```python
from build123d import *

# Parameters (mm, degrees)
SKETCH1_R           = 7
SKETCH1_R_2         = 4
BOSS_EXTRUDE1_DEPTH = 300
SKETCH2_R           = 5
CUT_EXTRUDE1_DEPTH  = 31
CUT_EXTRUDE2_START  = -269
SKETCH2_2_R         = 5
CUT_EXTRUDE2_DEPTH  = 31


with BuildPart() as part:
    # Sketch1 → Boss-Extrude1 (new body)
    with BuildSketch(Plane(origin=(0, 0, 0), x_dir=(1, 0, 0), z_dir=(0, 1, 0))):
        with Locations(Location((0, 0, 0), (0, 0, 270))):
            Circle(SKETCH1_R)
        with Locations(Location((0, 0, 0), (0, 0, 270))):
            Circle(SKETCH1_R_2, mode=Mode.SUBTRACT)
    extrude(amount=BOSS_EXTRUDE1_DEPTH)

    # Sketch2 → Cut-Extrude1 (cut)
    with BuildSketch(Plane(origin=(0, 300, 0), x_dir=(1, 0, 0), z_dir=(0, 1, 0))):
        with Locations(Location((0, 0, 0), (0, 0, 270))):
            Circle(SKETCH2_R)
    extrude(amount=-CUT_EXTRUDE1_DEPTH, mode=Mode.SUBTRACT)

    # Sketch2<2> → Cut-Extrude2 (cut)
    with BuildSketch(Plane(origin=(0, 300, 0), x_dir=(1, 0, 0), z_dir=(0, 1, 0)).offset(CUT_EXTRUDE2_START)):
        with Locations(Location((0, 0, 0), (0, 0, 270))):
            Circle(SKETCH2_2_R)
    extrude(amount=-CUT_EXTRUDE2_DEPTH, mode=Mode.SUBTRACT)


solid = part.part
```
Check sheet for the modelled part. Datum: model origin and axes. Units: mm. A direction names the side the tool comes from. Coordinates: 2 decimals unless noted, no trailing zeros. Order: outer loops, then holes, each group sorted by start corner. A loop starts at its lowest first (then second) coordinate and runs counter-clockwise, first axis right, second up. Notation, with made-up numbers: M -1,-2 L 25,-2 A14 ccw 25,12 Z; hole C -3,42.5 d5. An arc over 180 degrees is marked long. Write each question's results on one line, items separated by ' | '. Start each with the question number.
1. Go/stop test with flat-tipped pins: P1, Ø4, axis at y = 59.5, z = 2, coming from the -X side; P2, Ø6, axis at x = 0, z = 0, coming from the +Y side; P3, Ø4, axis at x = 3, y = 115, coming from the +Z side; P4, Ø6, axis at x = 5.5, y = 97, coming from the +Z side. Record where each tip stops, or that it passes through.
2. Cross-section at B-B on x = 0. Record the cut outline in (y, z), and give its area (3 significant figures).
3. Mould release check, pull along Z, two halves, no side actions. Record for faces 4 (the face through (-6.834, 147.9, -1.517)), 5 (the face through (5, 300, -2)), 6 (the face through (-3.905, 148.334, -0.867)): +Z half, -Z half, draft (parallel to the pull), parting line (faces both ways), or undercut.
4. Access from +Z, -Z, +X, -X, +Y, -Y to the whole of each face (thin tool, end or side, straight path). Record for faces 1 (the face through (-4.88, 15.72, -1.08)), 2 (the face through (-4.88, 284.72, -1.08)), 3 (the face through (5, 0, -2)).
5. Cross-section at C-C on y = 222.5. Record the cut outline in (x, z).
6. Material ranges on probe 1 along X at (y, z) = (287, 0); probe 2 along X at (y, z) = (103.5, 0); probe 3 along Y at (x, z) = (4, -1.75), recorded low to high.
7. Cross-section at A-A on z = 0. Record the cut outline in (x, y), and give its area (3 significant figures).
Checks:
1) P1: stops at x = -7 | P2: passes through | P3: stops at z = 6.93 | P4: stops at z = 6.54
2) outline: M 0,-7 L 300,-7 L 300,-5 L 269,-5 L 269,-4 L 31,-4 L 31,-5 L 0,-5 Z; M 0,5 L 31,5 L 31,4 L 269,4 L 269,5 L 300,5 L 300,7 L 0,7 Z | area: 1,680 mm²
3) face 4: parting line | face 5: draft | face 6: undercut
4) face 1: -Y | face 2: +Y | face 3: +Z, -Z, +X, -X, -Y
5) outline: C 0,0 d14; hole C 0,0 d8
6) probe 1: x = -7 to -5, 5 to 7 | probe 2: x = -7 to -4, 4 to 7 | probe 3: y = 31 to 269
7) outline: M -7,0 L -5,0 L -5,31 L -4,31 L -4,269 L -5,269 L -5,300 L -7,300 Z; M 4,31 L 5,31 L 5,0 L 7,0 L 7,300 L 5,300 L 5,269 L 4,269 Z | area: 1,680 mm²
